```python
from build123d import *

# Parameters (mm, degrees)
SKETCH_R        = 6
PAD_DEPTH       = 6
SKETCH001_R     = 1.75
POCKET_DEPTH    = 6.001
POCKET001_DEPTH = 3.5
CHAMFER_SIZE    = 1


with BuildPart() as part:
    # Sketch → Pad (new body)
    with BuildSketch(Plane.XY):
        Circle(SKETCH_R)
    extrude(amount=PAD_DEPTH)

    # Sketch001 → Pocket (cut, through all)
    with BuildSketch(Plane.XY.offset(6)):
        Circle(SKETCH001_R)
    extrude(amount=-POCKET_DEPTH, mode=Mode.SUBTRACT)

    # Sketch002 → Pocket001 (cut)
    with BuildSketch(Plane.XY.offset(6)):
        Polygon((2.144846, -2.341574), (3.100286, 0.686704), (0.95544, 3.028278), (-2.144846, 2.341574), (-3.100286, -0.686704), (-0.95544, -3.028278), align=None)
    extrude(amount=-POCKET001_DEPTH, mode=Mode.SUBTRACT)

    # Chamfer
    chamfer_edges = [part.edges().sort_by_distance(p)[0] for p in [
        (-6, 0, 0),
    ]]
    chamfer(chamfer_edges, length=CHAMFER_SIZE)


solid = part.part
```
For this review, take the finished solid that the model builds, in its own axes (mm). A direction names the side the tool comes from. Give positions to 0.01 mm unless a question says otherwise; leave off trailing zeros. Loops run counter-clockwise (first coordinate to the right, second up) from the corner with the lowest first, then second, coordinate; pieces in that order, holes last. Notation, with made-up numbers: M -8.5,16.5 L 29.5,16.5 A13 ccw 29.5,23.5 Z; hole C 48.25,-32 d2. An arc over 180 degrees is marked long. One line per item, written item: value. Start each with the question number.
Q1. Add section D-D (z = 1.2). Give the boundary of the cut face in (x, y).
Q2. For L1, parallel to Y at x = 0, z = 1.9; L2, parallel to Z at x = 3, y = 0.75; L3, parallel to Y at x = 2, z = 5.7, list the stretches that pass through material, from the lowest coordinate up.
Q3. Add section A-A (z = 5.55). Give the boundary of the cut face in (x, y), and give its area (3 significant figures).
Q4. Add section B-B (x = 0). Give the boundary of the cut face in (y, z).
Q5. Draft analysis for pull direction X (two halves, no side actions). For faces 3 (the face through (-6, 0, 3)), 4 (the face through (3, -1, 6)), 5 (the face through (0.57, -2.69, 4.27)), state which applies: released by +X, released by -X, zero draft, split by the parting line, or undercut.
Q6. Machinability: for faces 1 (the face through (0, -2, 0)), 2 (the face through (2.616, -0.849, 4.274)), which of the approach directions +Z, -Z, +X, -X, +Y, -Y give a long, thin tool a straight path to every point of the face, cutting with its end or side? Answer none if there is none.
Q7. Add section C-C (y = 0). Give the boundary of the cut face in (x, z).
Q8. Clearance check with flat-ended pins moving along their axes: pin 1 Ø1.5 at (y, z) = (-4.5, 1.5) entering from +X; pin 2 Ø1 at (x, z) = (-2.5, 2.5) entering from +Y; pin 3 Ø3 at (x, y) = (0, -1) entering from +Z; pin 4 Ø6 at (x, y) = (-2, -4) entering from -Z. State where each tip first meets the part, or that it passes through.
Reply:
1. outline: C 0,0 d12; hole C 0,0 d3.5
2. L1: -6 to -1.75, 1.75 to 6
2. L2: 0 to 2.5
2. L3: -5.66 to -2.37, 1.89 to 5.66
3. outline: C 0,0 d12; hole M -3.1,-0.69 L -0.96,-3.03 L 2.14,-2.34 L 3.1,0.69 L 0.96,3.03 L -2.14,2.34 Z
3. area: 86.9 mm²
4. outline: M -6,1 L -5,0 L -1.75,0 L -1.75,2.5 L -2.82,2.5 L -2.82,6 L -6,6 Z; M 1.75,0 L 5,0 L 6,1 L 6,6 L 2.82,6 L 2.82,2.5 L 1.75,2.5 Z
5. face 3: split by the parting line
5. face 4: zero draft
5. face 5: undercut
6. face 1: -Z, +X, -X, +Y, -Y
6. face 2: +Z
7. outline: M -6,1 L -5,0 L -1.75,0 L -1.75,2.5 L -2.88,2.5 L -2.88,6 L -6,6 Z; M 1.75,0 L 5,0 L 6,1 L 6,6 L 2.88,6 L 2.88,2.5 L 1.75,2.5 Z
8. pin 1: x = 4.68
8. pin 2: y = 5.66
8. pin 3: z = 2.5
8. pin 4: z = 0
